Input: part model. Units: mm. Frame: model coordinates. Coordinates: 2 decimals unless noted, no trailing zeros. Write each loop counter-clockwise with the first axis right and the second up, starting at its lowest first coordinate (ties: lowest second). Pieces come first, ordered by that corner, then holes.
from build123d import *

# Parameters (mm, degrees)
SKETCH1_R           = 200
SKETCH1_R_2         = 3.5
BOSS_EXTRUDE1_DEPTH = 10
SKETCH2_R           = 2.5
CUT_EXTRUDE1_DEPTH  = 11
SKETCH3_R           = 2.5
CUT_EXTRUDE2_DEPTH  = 11
SKETCH4_R           = 2.5
CUT_EXTRUDE3_DEPTH  = 11


with BuildPart() as part:
    # Sketch1 → Boss-Extrude1 (new body)
    with BuildSketch(Plane.XY):
        Circle(SKETCH1_R)
        Circle(SKETCH1_R_2, mode=Mode.SUBTRACT)
    extrude(amount=BOSS_EXTRUDE1_DEPTH)

    # Sketch2 → Cut-Extrude1 (cut, through all)
    with BuildSketch(Plane.XY.offset(10)):
        with Locations((37.34, 33.25)):
            Circle(SKETCH2_R)
        with Locations((45.86, 77.44)):
            Circle(SKETCH2_R)
    extrude(amount=-CUT_EXTRUDE1_DEPTH, mode=Mode.SUBTRACT)

    # Sketch3 → Cut-Extrude2 (cut, through all)
    with BuildSketch(Plane.XY.offset(10)):
        with Locations((-18.71, -64.86)):
            Circle(SKETCH3_R)
    extrude(amount=-CUT_EXTRUDE2_DEPTH, mode=Mode.SUBTRACT)

    # Sketch4 → Cut-Extrude3 (cut, through all)
    with BuildSketch(Plane.XY.offset(10)):
        with Locations((82.82, -146.05)):
            Circle(SKETCH4_R)
    extrude(amount=-CUT_EXTRUDE3_DEPTH, mode=Mode.SUBTRACT)


solid = part.part
Item 1: Pin query (flat end, axial travel): pin 1 Ø4 at (x, z) = (73, 3.5) entering from -Y; pin 2 Ø5 at (x, z) = (12.5, 7.5) entering from -Y; pin 3 Ø8 at (x, y) = (-18.71, -64.86) entering from -Z; pin 4 Ø1.5 at (y, z) = (-92.5, 6) entering from -X. Return the tip coordinate at first contact, or that it passes through.
Item 2: Material intervals for line 1 (Y direction, x = 0, z = 3); line 2 (X direction, y = -6, z = 5.25); line 3 (X direction, y = -146.05, z = 4.75), sorted ascending.
Item 3: Section query C-C, the plane x = -89.5. Return loops of the section in (y, z), then the cut area to 3 significant figures.
Item 4: Section query B-B, the plane y = 147. Return loops of the section in (x, z).
Item 5: Section query A-A, the plane z = 8.25. Return loops of the section in (x, y).
The answers:
1. pin 1: stops at y = -186.97
1. pin 2: stops at y = -199.75
1. pin 3: stops at z = 0
1. pin 4: stops at x = -177.71
2. line 1: y = -200 to -3.5, 3.5 to 200
2. line 2: x = -199.91 to 199.91
2. line 3: x = -136.64 to 80.32, 85.32 to 136.64
3. outline: (-178.86, 0) - (178.86, 0) - (178.86, 10) - (-178.86, 10) - close
3. area: 3,580 mm2
4. outline: (-135.61, 0) - (135.61, 0) - (135.61, 10) - (-135.61, 10) - close
5. outline: circle Ø400 at (0, 0); hole circle Ø5 at (-18.71, -64.86); hole circle Ø7 at (0, 0); hole circle Ø5 at (37.34, 33.25); hole circle Ø5 at (45.86, 77.44); hole circle Ø5 at (82.82, -146.05)
